Could you check a few things on this model? Use its own coordinates, in mm. Face numbers are marked on the shaded views. A direction names the side the tool comes from. Round coordinates to 2 decimals unless told otherwise and drop trailing zeros. Loops run counter-clockwise (first coordinate to the right, second up) from the corner with the lowest first, then second, coordinate; pieces in that order, holes last. Notation, with made-up numbers: (-40, -36) -> (-5, -36) arc R8 ccw to (-5, -27) -> close; hole circle Ø11 at (10, 45.5). An arc over 180 degrees is marked (long way). Write each question's results on one line, items separated by ' | '.
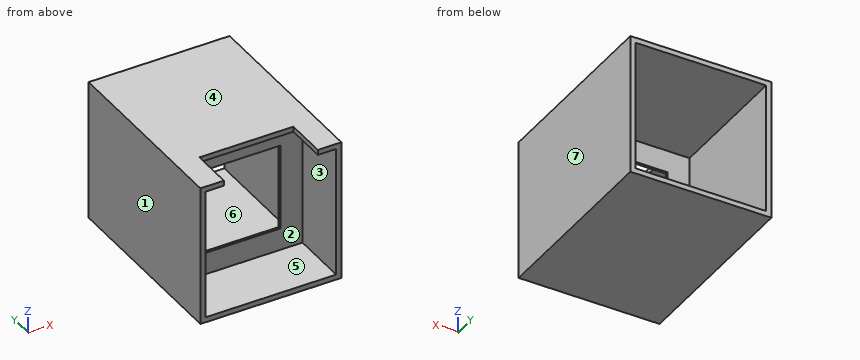
from build123d import *

# Parameters (mm, degrees)
SKETCH1_W           = 54
SKETCH1_H           = 54
SKETCH1_W_2         = 50
SKETCH1_H_2         = 50
BOSS_EXTRUDE1_DEPTH = 22
SKETCH2_W           = 54
SKETCH2_H           = 54
BOSS_EXTRUDE2_DEPTH = 1
SKETCH3_R           = 6
CUT_EXTRUDE1_DEPTH  = 24
SKETCH4_W           = 2
SKETCH4_H           = 50
SKETCH4_H_2         = 2
SKETCH4_W_2         = 50
BOSS_EXTRUDE3_DEPTH = 50
SKETCH5_W           = 33
SKETCH5_H           = 33
CUT_EXTRUDE2_DEPTH  = 52
CUT_EXTRUDE3_REACH  = 56
SKETCH6_W           = 36
SKETCH6_H           = 16


with BuildPart() as part:
    # Sketch1 → Boss-Extrude1 (new body)
    with BuildSketch(Plane(origin=(0, 0, 0), x_dir=(1, 0, 0), z_dir=(0, 1, 0))):
        Rectangle(SKETCH1_W, SKETCH1_H)
        Rectangle(SKETCH1_W_2, SKETCH1_H_2, mode=Mode.SUBTRACT)
    extrude(amount=BOSS_EXTRUDE1_DEPTH)

    # Sketch2 → Boss-Extrude2 (add)
    with BuildSketch(Plane(origin=(0, 22, 0), x_dir=(1, 0, 0), z_dir=(0, 1, 0))):
        Rectangle(SKETCH2_W, SKETCH2_H)
    extrude(amount=BOSS_EXTRUDE2_DEPTH)

    # Sketch3 → Cut-Extrude1 (cut, through all)
    with BuildSketch(Plane(origin=(0, 23, 0), x_dir=(1, 0, 0), z_dir=(0, 1, 0))):
        Circle(SKETCH3_R)
    extrude(amount=-CUT_EXTRUDE1_DEPTH, mode=Mode.SUBTRACT)

    # Sketch4 → Boss-Extrude3 (add)
    with BuildSketch(Plane(origin=(0, 23, 0), x_dir=(1, 0, 0), z_dir=(0, 1, 0))):
        with Locations((-26, 0)):
            Rectangle(SKETCH4_W, SKETCH4_H)
        with Locations((-26, -26)):
            Rectangle(SKETCH4_W, SKETCH4_H_2)
        with Locations((0, -26)):
            Rectangle(SKETCH4_W_2, SKETCH4_H_2)
        with Locations((26, -26)):
            Rectangle(SKETCH4_W, SKETCH4_H_2)
        with Locations((26, 0)):
            Rectangle(SKETCH4_W, SKETCH4_H)
        with Locations((26, 26)):
            Rectangle(SKETCH4_W, SKETCH4_H_2)
        with Locations((0, 26)):
            Rectangle(SKETCH4_W_2, SKETCH4_H_2)
        with Locations((-26, 26)):
            Rectangle(SKETCH4_W, SKETCH4_H_2)
    extrude(amount=BOSS_EXTRUDE3_DEPTH)

    # Sketch5 → Cut-Extrude2 (cut, through all)
    with BuildSketch(Plane.XZ.offset(-22)):
        Rectangle(SKETCH5_W, SKETCH5_H)
    extrude(amount=-CUT_EXTRUDE2_DEPTH, mode=Mode.SUBTRACT)

    # Sketch6 → Cut-Extrude3 (cut, up to next)
    with BuildSketch(Plane.XY.offset(27), mode=Mode.PRIVATE) as cut_extrude3_sk1:
        with Locations((0, 8)):
            Rectangle(SKETCH6_W, SKETCH6_H)
    cut_extrude3_tool1 = extrude(cut_extrude3_sk1.sketch, amount=-CUT_EXTRUDE3_REACH, mode=Mode.PRIVATE) & part.part
    add(cut_extrude3_tool1.solids().sort_by_distance((0, 8, 27))[0], mode=Mode.SUBTRACT)


solid = part.part
1) I want a section at A-A, the plane x = -15. Write out the boundary of the cut face in (y, z), plus the area to 3 significant figures.
Model answer:
outline: (0, -27) -> (73, -27) -> (73, -25) -> (23, -25) -> (23, -16.5) -> (22, -16.5) -> (22, -25) -> (0, -25) -> close; (16, 25) -> (22, 25) -> (22, 16.5) -> (23, 16.5) -> (23, 25) -> (73, 25) -> (73, 27) -> (16, 27) -> close | area: 277 mm2
2) I'm going to push flat-ended pins straight in: pin 1 (3 mm diameter, centred on x = 14.5, z = 11.5, fed in from +Y); pin 2 (25 mm diameter, centred on x = -4, z = 7, fed in from -Y); pin 3 (25 mm diameter, centred on x = -8.5, z = 2, fed in from +Y); pin 4 (2 mm diameter, centred on x = 2.5, z = 25.5, fed in from -Y). Where does each tip first touch, or does it pass through?
Model answer:
pin 1: passes through | pin 2: stops at y = 22 | pin 3: stops at y = 23 | pin 4: stops at y = 16
3) I need wall thicknesses on line 1 (Z direction, x = -12, y = 30.5); line 2 (Z direction, x = -13.5, y = 12). Which ranges of each line are inside material? Lowest first, please.
Model answer:
line 1: z = -27 to -25, 25 to 27 | line 2: z = -27 to -25
4) If we mould it in two halves opening along Z, with no side actions, what happens to the marked faces 1, 2, 3 and 4? For each: released by +Z, released by -Z, zero draft, split by the parting line, or undercut.
Model answer:
face 1: zero draft | face 2: undercut | face 3: undercut | face 4: released by +Z
5) For the marked faces 5, 6 and 7, which set-ups out of +Z, -Z, +X, -X, +Y, -Y let a thin tool reach every point of the face, with its end or its side?
Model answer:
face 5: -Y | face 6: +Y | face 7: +Z, -Z, +X, +Y, -Y
6) I want a section at D-D, the plane z = -23. Write out the boundary of the cut face in (x, y).
Model answer:
outline: (-27, 0) -> (-25, 0) -> (-25, 22) -> (25, 22) -> (25, 0) -> (27, 0) -> (27, 73) -> (25, 73) -> (25, 23) -> (-25, 23) -> (-25, 73) -> (-27, 73) -> close
7) I want a section at C-C, the plane y = 26. Write out the boundary of the cut face in (x, z), plus the area to 3 significant figures.
Model answer:
outline: (-27, -27) -> (27, -27) -> (27, 27) -> (-27, 27) -> close; hole (-25, -25) -> (25, -25) -> (25, 25) -> (-25, 25) -> close | area: 416 mm2
8) I want a section at B-B, the plane z = -15. Write out the boundary of the cut face in (x, y).
Model answer:
outline: (-27, 0) -> (-25, 0) -> (-25, 22) -> (-16.5, 22) -> (-16.5, 23) -> (-25, 23) -> (-25, 73) -> (-27, 73) -> close; (16.5, 22) -> (25, 22) -> (25, 0) -> (27, 0) -> (27, 73) -> (25, 73) -> (25, 23) -> (16.5, 23) -> close
